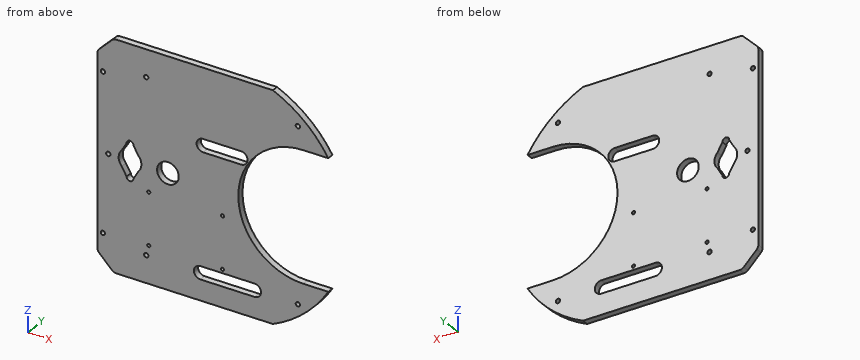
```python
from build123d import *

# Parameters (mm, degrees)
SKETCH1_R           = 2
SKETCH1_R_2         = 10.5
BOSS_EXTRUDE1_DEPTH = 6
SKETCH2_R           = 10
SKETCH2_R_2         = 2
CUT_EXTRUDE2_DEPTH  = 19
BOSS_EXTRUDE2_DEPTH = 6
CHAMFER1_SIZE       = 15
FILLET1_R           = 5
SKETCH4_R           = 1.5
CUT_EXTRUDE3_DEPTH  = 10
SKETCH5_R           = 2
CUT_EXTRUDE4_DEPTH  = 10


with BuildPart() as part:
    # Sketch1 → Boss-Extrude1 (new body)
    with BuildSketch(Plane(origin=(0, 0, 0), x_dir=(1, 0, 0), z_dir=(0, 1, 0))):
        with BuildLine():
            Line((-46.904157598, -105), (46.904157598, -105))
            ThreePointArc((46.904157598, -105), (115, 0), (46.904157598, 105))
            Line((46.904157598, 105), (-46.904157598, 105))
            ThreePointArc((-46.904157598, 105), (-115, 0), (-46.904157598, -105))
        make_face()
        with Locations((-70, 80)):
            Circle(SKETCH1_R, mode=Mode.SUBTRACT)
        with Locations((70, 80)):
            Circle(SKETCH1_R, mode=Mode.SUBTRACT)
        with Locations((70, -80)):
            Circle(SKETCH1_R, mode=Mode.SUBTRACT)
        with Locations((-70, -80)):
            Circle(SKETCH1_R, mode=Mode.SUBTRACT)
        with Locations((-85, 0)):
            Circle(SKETCH1_R_2, mode=Mode.SUBTRACT)
    extrude(amount=BOSS_EXTRUDE1_DEPTH)

    # Sketch2 → Cut-Extrude2 (cut)
    with BuildSketch(Plane.XZ):
        with Locations((-50, 0)):
            Circle(SKETCH2_R)
        with Locations((-105, 0)):
            Circle(SKETCH2_R_2)
        with BuildLine():
            Line((-88.153729078, 15), (-92.680195826, 7.159929613))
            ThreePointArc((-92.680195826, 7.159929613), (-95.5, 0), (-92.680195826, -7.159929613))
            Line((-92.680195826, -7.159929613), (-88.153729078, -15))
            ThreePointArc((-88.153729078, -15), (-85, -18.153729078), (-81.846270922, -15))
            Line((-81.846270922, -15), (-77.319804174, -7.159929613))
            ThreePointArc((-77.319804174, -7.159929613), (-74.5, 0), (-77.319804174, 7.159929613))
            Line((-77.319804174, 7.159929613), (-81.846270922, 15))
            ThreePointArc((-81.846270922, 15), (-85, 18.153729078), (-88.153729078, 15))
        make_face()
        with BuildLine():
            Line((-20, -74), (30, -74))
            ThreePointArc((30, -74), (36, -80), (30, -86))
            Line((30, -86), (-20, -86))
            ThreePointArc((-20, -86), (-26, -80), (-20, -74))
        make_face()
        with BuildLine():
            Line((17.5, 29), (-17.5, 29))
            ThreePointArc((-17.5, 29), (-23.5, 35), (-17.5, 41))
            Line((-17.5, 41), (17.5, 41))
            ThreePointArc((17.5, 41), (23.5, 35), (17.5, 29))
        make_face()
    extrude(amount=-CUT_EXTRUDE2_DEPTH, mode=Mode.SUBTRACT)

    # Sketch3 → Boss-Extrude2 (add)
    with BuildSketch(Plane(origin=(0, 0, 0), x_dir=(-1, 0, 0), z_dir=(0, -1, 0))):
        with BuildLine():
            ThreePointArc((115, 0), (96.485693561, -62.574043645), (46.904157598, -105))
            Line((46.904157598, -105), (115, -105))
            Line((115, -105), (115, 0))
        make_face()
        with BuildLine():
            ThreePointArc((46.904157598, 105), (96.485693561, 62.574043645), (115, 0))
            Line((115, 0), (115, 105))
            Line((115, 105), (46.904157598, 105))
        make_face()
    extrude(amount=-BOSS_EXTRUDE2_DEPTH)

    # Chamfer1
    chamfer1_edges = [part.edges().sort_by_distance(p)[0] for p in [
        (-115, 3, 105),
        (-115, 3, -105),
    ]]
    chamfer(chamfer1_edges, length=CHAMFER1_SIZE)

    # Fillet1
    fillet1_edges = [part.edges().sort_by_distance(p)[0] for p in [
        (-115, 3, 90),
        (-115, 3, -90),
        (-100, 3, -105),
        (-100, 3, 105),
    ]]
    fillet(fillet1_edges, radius=FILLET1_R)

    # Sketch4 → Cut-Extrude3 (cut)
    with BuildSketch(Plane(origin=(0, 6, 0), x_dir=(1, 0, 0), z_dir=(0, 1, 0))):
        with Locations((0.319804174, 22.536233459)):
            Circle(SKETCH4_R)
        with Locations((-67.680195826, 22.536233459)):
            Circle(SKETCH4_R)
        with Locations((-67.680195826, 70.536233459)):
            Circle(SKETCH4_R)
        with Locations((0.319804174, 70.536233459)):
            Circle(SKETCH4_R)
        with BuildLine():
            Line((115, -60), (75, -60))
            ThreePointArc((75, -60), (15, 0), (75, 60))
            Line((75, 60), (115, 60))
            Line((115, 60), (115, -60))
        make_face()
    extrude(amount=-CUT_EXTRUDE3_DEPTH, mode=Mode.SUBTRACT)

    # Sketch5 → Cut-Extrude4 (cut)
    with BuildSketch(Plane(origin=(0, 6, 0), x_dir=(1, 0, 0), z_dir=(0, 1, 0))):
        with Locations((-110, -72.5)):
            Circle(SKETCH5_R)
        with Locations((-110, 72.5)):
            Circle(SKETCH5_R)
    extrude(amount=-CUT_EXTRUDE4_DEPTH, mode=Mode.SUBTRACT)


solid = part.part
```
Source: CAD feature listing. Evaluate the final solid. Frame: model axes, mm. Coordinates: 2 decimals unless noted, no trailing zeros. Write each loop counter-clockwise with the first axis right and the second up, starting at its lowest first coordinate (ties: lowest second). Pieces come first, ordered by that corner, then holes. Notation, with made-up numbers: M 67.5,72.5 L 109.5,72.5 A15 cw 109.5,101.5 Z; hole C -18.5,72.5 d1. An arc over 180 degrees is marked long. Answer as a JSON object with one key per item and string values.
1. Cut plane C-C on z = -47.5. Output: boundary loops of the cut face in (x, y), plus the area to 3 significant figures.
Evaluation:
{"outline": "M -115,0 L 38.34,0 L 38.34,6 L -115,6 Z", "area": "920 mm^2"}
2. Contact query for flat-ended pins moving along their axis: P1, Ø4.5, axis at x = -70, z = 80, coming from the +Y side; P2, Ø2.5, axis at x = 0.32, z = -22.54, coming from the -Y side; P3, Ø2, axis at y = 1, z = -31, coming from the +X side. Output: stop coordinate, or through.
Evaluation:
{"P1": "y = 6", "P2": "through", "P3": "x = 24.25"}
3. Cut plane D-D on y = 3.8. State how many separate pieces and enclosed holes the cut face has, plus the area to 3 significant figures.
Evaluation:
{"separate pieces": "1", "enclosed holes": "15", "area": "32,100 mm^2"}
4. Cut plane B-B on x = 83. Output: boundary loops of the cut face in (y, z).
Evaluation:
{"outline": "M 0,-79.6 L 6,-79.6 L 6,-60 L 0,-60 Z; M 0,60 L 6,60 L 6,79.6 L 0,79.6 Z"}
5. Ray query, L1, parallel to Z at x = -7, y = 1.85; L2, parallel to Z at x = 0, y = 1.75; L3, parallel to X at y = 4.75, z = -80. Return the intervals inside material, ascending.
Evaluation:
{"L1": "-105 to -86, -74 to 29, 41 to 105", "L2": "-105 to -86, -74 to -72, -69.07 to -24, -21.07 to 29, 41 to 105", "L3": "-115 to -72, -68 to -26, 36 to 68, 72 to 82.61"}
6. Cut plane A-A on x = -50. Output: boundary loops of the cut face in (y, z), plus the area to 3 significant figures.
Evaluation:
{"outline": "M 0,-105 L 6,-105 L 6,-10 L 0,-10 Z; M 0,10 L 6,10 L 6,105 L 0,105 Z", "area": "1,140 mm^2"}
